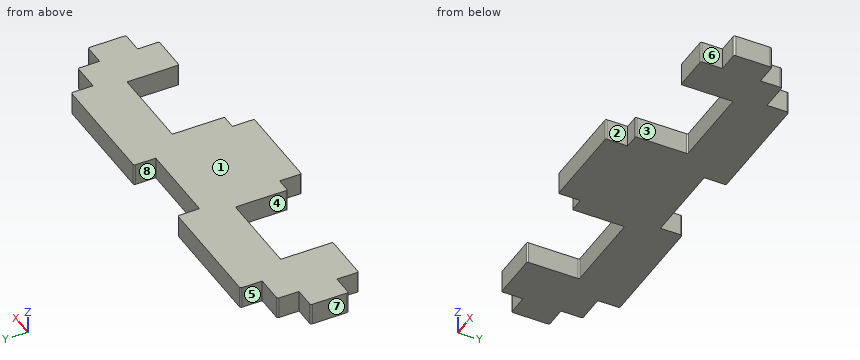
from build123d import *

# Parameters (mm, degrees)
BOSS_EXTRUDE1_DEPTH = 3


with BuildPart() as part:
    # Sketch2 → Boss-Extrude1 (new body)
    with BuildSketch(Plane.XY):
        with BuildLine():
            Line((53.652188988, 7.790592853), (53.652188988, 4.988083366))
            ThreePointArc((53.652188988, 4.988083366), (53.60349827, 4.870533572), (53.485948476, 4.821842853))
            Line((53.485948476, 4.821842853), (48.668429501, 4.821842853))
            ThreePointArc((48.668429501, 4.821842853), (48.550879707, 4.870533572), (48.502188988, 4.988083366))
            Line((48.502188988, 4.988083366), (48.502188988, 11.80560234))
            ThreePointArc((48.502188988, 11.80560234), (48.45349827, 11.923152134), (48.335948476, 11.971842853))
            Line((48.335948476, 11.971842853), (36.968429501, 11.971842853))
            ThreePointArc((36.968429501, 11.971842853), (36.850879707, 11.923152134), (36.802188988, 11.80560234))
            Line((36.802188988, 11.80560234), (36.802188988, 4.988083366))
            ThreePointArc((36.802188988, 4.988083366), (36.75349827, 4.870533572), (36.635948476, 4.821842853))
            Line((36.635948476, 4.821842853), (34.752188988, 4.821842853))
            Line((34.752188988, 4.821842853), (34.752188988, 1.988083366))
            ThreePointArc((34.752188988, 1.988083366), (34.70349827, 1.870533572), (34.585948476, 1.821842853))
            Line((34.585948476, 1.821842853), (22.718429501, 1.821842853))
            ThreePointArc((22.718429501, 1.821842853), (22.600879707, 1.870533572), (22.552188988, 1.988083366))
            Line((22.552188988, 1.988083366), (22.552188988, 4.821842853))
            Line((22.552188988, 4.821842853), (20.668429501, 4.821842853))
            ThreePointArc((20.668429501, 4.821842853), (20.550879707, 4.870533572), (20.502188988, 4.988083366))
            Line((20.502188988, 4.988083366), (20.502188988, 11.80560234))
            ThreePointArc((20.502188988, 11.80560234), (20.45349827, 11.923152134), (20.335948476, 11.971842853))
            Line((20.335948476, 11.971842853), (8.968429501, 11.971842853))
            ThreePointArc((8.968429501, 11.971842853), (8.850879707, 11.923152134), (8.802188988, 11.80560234))
            Line((8.802188988, 11.80560234), (8.802188988, 4.988083366))
            ThreePointArc((8.802188988, 4.988083366), (8.75349827, 4.870533572), (8.635948476, 4.821842853))
            Line((8.635948476, 4.821842853), (2.318429501, 4.821842853))
            ThreePointArc((2.318429501, 4.821842853), (2.200879707, 4.870533572), (2.152188988, 4.988083366))
            Line((2.152188988, 4.988083366), (2.152188988, 7.790592853))
            Line((2.152188988, 7.790592853), (-0.597811012, 7.790592853))
            ThreePointArc((-0.597811012, 7.790592853), (-0.774587707, 7.863816157), (-0.847811012, 8.040592853))
            Line((-0.847811012, 8.040592853), (-0.847811012, 12.740592853))
            ThreePointArc((-0.847811012, 12.740592853), (-0.774587707, 12.917369548), (-0.597811012, 12.990592853))
            Line((-0.597811012, 12.990592853), (2.152188988, 12.990592853))
            Line((2.152188988, 12.990592853), (2.152188988, 15.709342853))
            ThreePointArc((2.152188988, 15.709342853), (2.225412293, 15.886119548), (2.402188988, 15.959342853))
            Line((2.402188988, 15.959342853), (6.052188988, 15.959342853))
            Line((6.052188988, 15.959342853), (6.052188988, 18.709342853))
            ThreePointArc((6.052188988, 18.709342853), (6.125412293, 18.886119548), (6.302188988, 18.959342853))
            Line((6.302188988, 18.959342853), (22.002188988, 18.959342853))
            ThreePointArc((22.002188988, 18.959342853), (22.178965684, 18.886119548), (22.252188988, 18.709342853))
            Line((22.252188988, 18.709342853), (22.252188988, 15.959342853))
            Line((22.252188988, 15.959342853), (33.552188988, 15.959342853))
            Line((33.552188988, 15.959342853), (33.552188988, 18.709342853))
            ThreePointArc((33.552188988, 18.709342853), (33.625412293, 18.886119548), (33.802188988, 18.959342853))
            Line((33.802188988, 18.959342853), (49.502188988, 18.959342853))
            ThreePointArc((49.502188988, 18.959342853), (49.678965684, 18.886119548), (49.752188988, 18.709342853))
            Line((49.752188988, 18.709342853), (49.752188988, 15.959342853))
            Line((49.752188988, 15.959342853), (53.402188988, 15.959342853))
            ThreePointArc((53.402188988, 15.959342853), (53.578965684, 15.886119548), (53.652188988, 15.709342853))
            Line((53.652188988, 15.709342853), (53.652188988, 12.990592853))
            Line((53.652188988, 12.990592853), (56.402188988, 12.990592853))
            ThreePointArc((56.402188988, 12.990592853), (56.578965684, 12.917369548), (56.652188988, 12.740592853))
            Line((56.652188988, 12.740592853), (56.652188988, 8.040592853))
            ThreePointArc((56.652188988, 8.040592853), (56.578965684, 7.863816157), (56.402188988, 7.790592853))
            Line((56.402188988, 7.790592853), (53.652188988, 7.790592853))
        make_face()
    extrude(amount=BOSS_EXTRUDE1_DEPTH)


solid = part.part
CAD build for the part. Positions are in the model's coordinates, mm. Face numbers are marked on the shaded views. A direction names the side the tool comes from. Round coordinates to 2 decimals unless told otherwise and drop trailing zeros. Loops run counter-clockwise (first coordinate to the right, second up) from the corner with the lowest first, then second, coordinate; pieces in that order, holes last.
(1) Cut at B-B (y = 8.75). Give the cut face in (x, z).
(2) Cut at C-C (x = 10). Give the cut face in (y, z), plus the area to 3 significant figures.
(3) Wall check: line 1 along X through (y, z) = (11, 0.45); line 2 along X through (y, z) = (5.25, 2.75); line 3 along X through (y, z) = (17, 2.6). Give the ranges that are in metal, low to high.
(4) Cut at D-D (x = 29.5). Give the cut face in (y, z), plus the area to 3 significant figures.
(5) Which spindle directions (+Z, -Z, +X, -X, +Y, -Y) get a long thin tool onto all of the face, cutting with end or side? Do the marked faces 4, 5, 6, 7 and 8. Say none if no direction does.
(6) Drop flat-ended pins along their axis: pin 1 (0.9 mm diameter, centred on x = 52.5, z = 2, fed in from +Y); pin 2 (0.8 mm diameter, centred on y = 17, z = 1, fed in from +X); pin 3 (0.9 mm diameter, centred on x = 36, z = 1.5, fed in from -Y). Give the stop position or say it passes through.
(7) Cut at A-A (y = 16.75). Give the cut face in (x, z), plus the area to 3 significant figures.
(8) Two-plate mould, pull along X, no slides. Class the marked faces 1, 2 and 3: +X half, -X half, draft (parallel to the pull), parting line (faces both ways), or undercut.
Findings below:
1. outline: (-0.85, 0) - (8.8, 0) - (8.8, 3) - (-0.85, 3) - close; (20.5, 0) - (36.8, 0) - (36.8, 3) - (20.5, 3) - close; (48.5, 0) - (56.65, 0) - (56.65, 3) - (48.5, 3) - close
2. outline: (11.97, 0) - (18.96, 0) - (18.96, 3) - (11.97, 3) - close
2. area: 21.0 mm2
3. line 1: x = -0.85 to 8.8, 20.5 to 36.8, 48.5 to 56.65
3. line 2: x = 2.15 to 8.8, 20.5 to 36.8, 48.5 to 53.65
3. line 3: x = 6.05 to 22.25, 33.55 to 49.75
4. outline: (1.82, 0) - (15.96, 0) - (15.96, 3) - (1.82, 3) - close
4. area: 42.4 mm2
5. face 4: +Z, -Z, -Y
5. face 5: +Z, -Z, -X, +Y
5. face 6: +Z, -Z, +X, -Y
5. face 7: +Z, -Z, -X, +Y, -Y
5. face 8: +Z, -Z, +Y
6. pin 1: stops at y = 15.96
6. pin 2: stops at x = 49.75
6. pin 3: stops at y = 4.82
7. outline: (6.05, 0) - (22.25, 0) - (22.25, 3) - (6.05, 3) - close; (33.55, 0) - (49.75, 0) - (49.75, 3) - (33.55, 3) - close
7. area: 97.2 mm2
8. face 1: draft
8. face 2: +X half
8. face 3: undercut
